The model under review builds one solid part; all positions refer to its coordinate system, in mm. A direction names the side the tool comes from. Round coordinates to 2 decimals unless told otherwise and drop trailing zeros. Loops run counter-clockwise (first coordinate to the right, second up) from the corner with the lowest first, then second, coordinate; pieces in that order, holes last. Notation, with made-up numbers: (15, 18.5) -> (50, 18.5) arc R28 ccw to (50, 40.5) -> close; hole circle Ø7 at (39.5, 54). An arc over 180 degrees is marked (long way). Use a Markdown table: item, result. Add a question column.
1) Wall thickness on probe 1 along Y at (x, z) = (38.1, 49.9); probe 2 along X at (y, z) = (-29.5, 19); probe 3 along Z at (x, y) = (30.75, -81.5): over which ranges is each line inside the solid? List them lowest first.
2) For faces 1 (the cylindrical face through (40.561, -24.625, 49.856)), 2 (the flat face through (27.051, -50, 26)), list the 3-axis set-ups (+Z, -Z, +X, -X, +Y, -Y) from which the entire face can be reached by the end or side of a thin tool; tool diameter is ignored.
3) Mouldability with a two-part tool opening along Y and no side actions: class faces 3 (the cylindrical face through (39.487, -48.625, 0.707)), 4 (the flat face through (49.3, -88.9, 23.3)), 5 (the flat face through (41, -50, 49.019)) as released by +Y, released by -Y, zero draft, split by the parting line, or undercut.
4) Consider section B-B on x = 32.5. Give the boundary of the cut face in (y, z).
5) Consider section A-A on z = 17. Give the boundary of the cut face in (x, y), plus the area to 3 significant figures.
6) Consider section C-C on x = 38.1. Give the boundary of the cut face in (y, z).
7) Consider section D-D on y = -25.4. Give the boundary of the cut face in (x, z), plus the area to 3 significant figures.
Autodesk Inventor part; units mm, degrees
ref_plane "YZ Plane" through (0, 0, 0) normal (1, 0, 0) x (0, 1, 0)
ref_plane "XZ Plane" through (0, 0, 0) normal (0, 1, 0) x (-1, 0, 0)
ref_plane "XY Plane" through (0, 0, 0) normal (0, 0, 1) x (1, 0, 0)
ref_plane "Work Plane1" through (50.8, -12.7, 0) normal (0, -1, 0) x (0, 0, 1)
sketch "Sketch1" plane through (50.8, -12.7, 0) normal (0, -1, 0) x (0, 0, 1)
  line L0 (-0.1298, 0) -> (50.6702, 0)
  line L1 (50.6702, 0) -> (50.6702, 25.4)
  line L2 (50.6702, 25.4) -> (-0.1298, 25.4)
  line L3 (-0.1298, 25.4) -> (-0.1298, 0)
  line L4 (49.0192, 23.749) -> (1.5212, 23.749)
  line L5 (1.5212, 23.749) -> (1.5212, 1.651)
  line L6 (1.5212, 1.651) -> (49.0192, 1.651)
  line L7 (49.0192, 1.651) -> (49.0192, 23.749)
  point P0 (0, 50.8)
  dimension "d0" = 25.4
  dimension "d1" = 50.8
  dimension "d3" = 1.651
  dimension "d4" = 1.651
  dimension "d5" = 1.651
  dimension "d6" = 1.651
extrude "Extrusion1" add sketch "Sketch1" along normal blind 76.2
sketch "Sketch2" plane through (25.4, -12.7, 50.6702) normal (0, 0, 1) x (1, 0, 0)
  circle A0 centre (12.7, -12.7) radius 2.5797
  circle A1 centre (12.7, -38.1) radius 2.5797
  line L0 (25.4, 0) -> (0, 0)
  line L1 (0, 0) -> (0, -76.2)
  point P0 (-25.4, 12.7)
  dimension "d9" = 12.7
  dimension "d10" = 25.4
  dimension "d11" = 5.1594
  dimension "d12" = 5.1594
  dimension "d13" = 12.7
  dimension "d14" = 12.7
extrude "Extrusion2" cut sketch "Sketch2" against normal blind 76.2
equation "\"d4\" = d3"
equation "\"d5\" = d3"
equation "\"d6\" = d3"
properties part number "bar thing"
Result set:
| question | item | result |
|---|---|---|
| 1 | probe 1 | -88.9 to -53.38, -48.22 to -27.98, -22.82 to -12.7 |
| 1 | probe 2 | 25.4 to 27.05, 49.15 to 50.8 |
| 1 | probe 3 | -0.13 to 1.52, 49.02 to 50.67 |
| 2 | face 1 | +Z, -Z |
| 2 | face 2 | +Y, -Y |
| 3 | face 3 | undercut |
| 3 | face 4 | released by -Y |
| 3 | face 5 | zero draft |
| 4 | outline | (-88.9, -0.13) -> (-12.7, -0.13) -> (-12.7, 1.52) -> (-88.9, 1.52) -> close; (-88.9, 49.02) -> (-12.7, 49.02) -> (-12.7, 50.67) -> (-88.9, 50.67) -> close |
| 5 | outline | (25.4, -88.9) -> (27.05, -88.9) -> (27.05, -12.7) -> (25.4, -12.7) -> close; (49.15, -88.9) -> (50.8, -88.9) -> (50.8, -12.7) -> (49.15, -12.7) -> close |
| 5 | area | 252 mm2 |
| 6 | outline | (-88.9, -0.13) -> (-53.38, -0.13) -> (-53.38, 1.52) -> (-88.9, 1.52) -> close; (-88.9, 49.02) -> (-53.38, 49.02) -> (-53.38, 50.67) -> (-88.9, 50.67) -> close; (-48.22, -0.13) -> (-27.98, -0.13) -> (-27.98, 1.52) -> (-48.22, 1.52) -> close; (-48.22, 49.02) -> (-27.98, 49.02) -> (-27.98, 50.67) -> (-48.22, 50.67) -> close; (-22.82, -0.13) -> (-12.7, -0.13) -> (-12.7, 1.52) -> (-22.82, 1.52) -> close; (-22.82, 49.02) -> (-12.7, 49.02) -> (-12.7, 50.67) -> (-22.82, 50.67) -> close |
| 7 | outline | (25.4, -0.13) -> (35.52, -0.13) -> (35.52, 1.52) -> (27.05, 1.52) -> (27.05, 49.02) -> (35.52, 49.02) -> (35.52, 50.67) -> (25.4, 50.67) -> close; (40.68, -0.13) -> (50.8, -0.13) -> (50.8, 50.67) -> (40.68, 50.67) -> (40.68, 49.02) -> (49.15, 49.02) -> (49.15, 1.52) -> (40.68, 1.52) -> close |
| 7 | area | 224 mm2 |
